Can you work these out from the model? Positions are in its coordinate system, mm. A direction names the side the tool comes from. Give positions to 0.01 mm unless a question says otherwise; leave off trailing zeros. Loops run counter-clockwise (first coordinate to the right, second up) from the corner with the lowest first, then second, coordinate; pieces in that order, holes last. Notation, with made-up numbers: (-12.5, -4) - (11.5, -4) arc R26 ccw to (11.5, 27) - close; hole circle Ø11 at (78, 43.5). An arc over 180 degrees is marked (long way). Write item = value, one per line.
Autodesk Inventor part; units mm, degrees
ref_plane "YZ Plane" through (0, 0, 0) normal (1, 0, 0) x (0, 1, 0)
ref_plane "XZ Plane" through (0, 0, 0) normal (0, 1, 0) x (-1, 0, 0)
ref_plane "XY Plane" through (0, 0, 0) normal (0, 0, 1) x (1, 0, 0)
sketch "Sketch1" plane through (0, 0, 0) normal (0, 0, 1) x (1, 0, 0)
  circle A0 centre (0, 0) radius 7.2
  dimension "d0" = 14.4
extrude "Extrusion1" add sketch "Sketch1" along normal blind 16.5
sketch "Sketch2" plane through (0, 0, 16.5) normal (0, 0, 1) x (1, 0, 0)
  circle A0 centre (0, 0) radius 2.5
  dimension "d3" = 5
extrude "Extrusion2" cut sketch "Sketch2" against normal blind 10
sketch "Sketch5" plane through (0, 0, 0) normal (0, 0, -1) x (-1, 0, 0)
  line L0 (17.8427, 0) -> (-13.8887, 0)
  line L1 (-9.3556, 0) -> (13.3097, 0)
  line L2 (13.3097, 0) -> (13.3097, -11.7916)
  line L3 (13.3097, -11.7916) -> (-9.3556, -11.7916)
  line L4 (-9.3556, -11.7916) -> (-9.3556, 0)
  point P0 (0, 0)
extrude "Extrusion4" cut sketch "Sketch5" against normal up to surface (16.5 mm away)
properties part number "HoleFill4"
Q1. Imagine slicing it at B-B, the plane y = 1. Write out the boundary of the cut face in (x, z), then the cut area to 3 significant figures.
Output:
outline = (-7.13, 0) - (7.13, 0) - (7.13, 16.5) - (2.29, 16.5) - (2.29, 6.5) - (-2.29, 6.5) - (-2.29, 16.5) - (-7.13, 16.5) - close
area = 189 mm2
Q2. Imagine slicing it at C-C, the plane z = 11.5. Write out the boundary of the cut face in (x, y).
Output:
outline = (-7.2, 0) - (-2.5, 0) arc R2.5 cw to (2.5, 0) - (7.2, 0) arc R7.2 ccw to start
Q3. We'd pull the mould along X, two halves only. Please class faces 1 (the flat face through (0, 1, 6.5)), 2 (the cylindrical face through (-0.16, 7.2, 8.13)), 3 (the flat face through (0, 0, 6)): released by +X, released by -X, zero draft, split by the parting line, or undercut.
Output:
face_1 = undercut
face_2 = split by the parting line
face_3 = zero draft
Q4. Imagine slicing it at D-D, the plane y = 5.25. Write out the boundary of the cut face in (x, z), then the cut area to 3 significant figures.
Output:
outline = (-4.93, 0) - (4.93, 0) - (4.93, 16.5) - (-4.93, 16.5) - close
area = 163 mm2
Q5. For pin 1 (1 mm diameter, centred on y = 1, z = 2.5, fed in from -X); pin 2 (1.5 mm diameter, centred on y = 6, z = 10, fed in from -X); pin 3 (1.2 mm diameter, centred on x = -1, y = 1.5, fed in from +Z), each with a flat end and sliding along its axis, tell me the tip position at first contact or that it passes through.
Output:
pin_1 = -7.18
pin_2 = -4.93
pin_3 = 6.5
Q6. Which directions (+Z, -Z, +X, -X, +Y, -Y) give clear straight access to the entire face, cutting with the end or side of a thin tool? Please do faces 4 (the cylindrical face through (0.1, 2.5, 11.6)), 5 (the flat face through (0, 4, 16.5)).
Output:
face_4 = +Z, -Y
face_5 = +Z, +X, -X, +Y, -Y
Q7. I need wall thicknesses on L1, parallel to X at y = 1.25, z = 15.75; L2, parallel to X at y = 2, z = 10.5; L3, parallel to Z at x = -1.25, y = 2. Which ranges of each line are inside material? Lowest first, please.
Output:
L1 = -7.09 to -2.17, 2.17 to 7.09
L2 = -6.92 to -1.5, 1.5 to 6.92
L3 = 0 to 6.5
Q8. Imagine slicing it at A-A, the plane x = 0. Write out the boundary of the cut face in (y, z), then the cut area to 3 significant figures.
Output:
outline = (0, 0) - (7.2, 0) - (7.2, 16.5) - (2.5, 16.5) - (2.5, 6.5) - (0, 6.5) - close
area = 93.8 mm2
